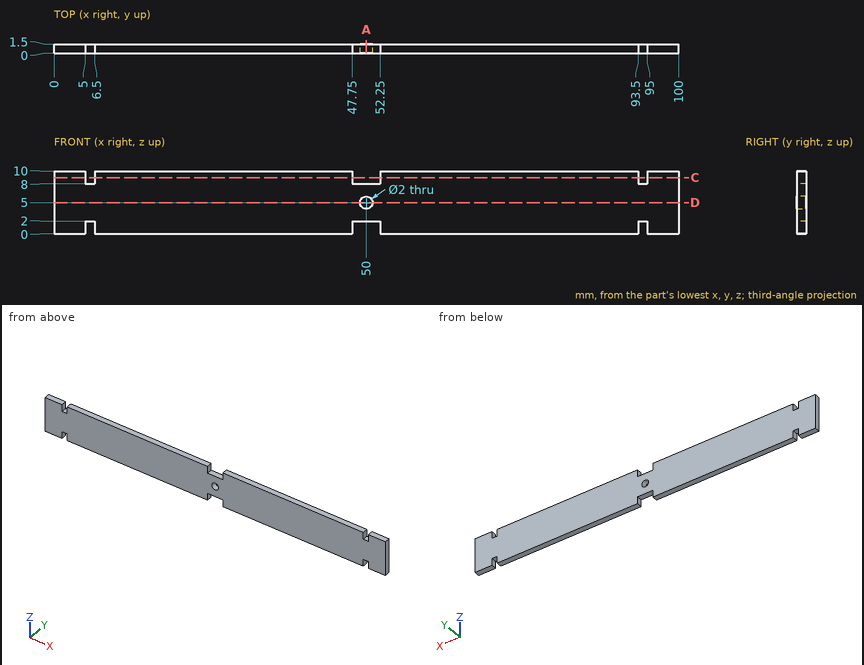
Source: three-view drawing plus pictorial views. Frame: mm from the lowest corner of the part. Round coordinates to 2 decimals unless told otherwise and drop trailing zeros. Loops run counter-clockwise (first coordinate to the right, second up) from the corner with the lowest first, then second, coordinate; pieces in that order, holes last.
Q1. Section A-A, the plane x = 50. Return loops of the section in (y, z), plus the area to 3 significant figures.
Q2. Section C-C, the plane z = 9. Return loops of the section in (x, y), plus the area to 3 significant figures.
Q3. Ray query, line 1 (X direction, y = 0.1, z = 0.5); line 2 (Z direction, x = 50, y = 0.7); line 3 (X direction, y = 0.5, z = 5). Return the intervals inside material, ascending.
Q4. Section D-D, the plane z = 5. Return loops of the section in (x, y), plus the area to 3 significant figures.
Solutions:
1. outline: (0, 2) - (1.5, 2) - (1.5, 4) - (0, 4) - close; (0, 6) - (1.5, 6) - (1.5, 8) - (0, 8) - close
1. area: 6.00 mm2
2. outline: (0, 0) - (5, 0) - (5, 1.5) - (0, 1.5) - close; (6.5, 0) - (47.75, 0) - (47.75, 1.5) - (6.5, 1.5) - close; (52.25, 0) - (93.5, 0) - (93.5, 1.5) - (52.25, 1.5) - close; (95, 0) - (100, 0) - (100, 1.5) - (95, 1.5) - close
2. area: 139 mm2
3. line 1: x = 0 to 5, 6.5 to 47.75, 52.25 to 93.5, 95 to 100
3. line 2: z = 2 to 4, 6 to 8
3. line 3: x = 0 to 49, 51 to 100
4. outline: (0, 0) - (49, 0) - (49, 1.5) - (0, 1.5) - close; (51, 0) - (100, 0) - (100, 1.5) - (51, 1.5) - close
4. area: 147 mm2
